from build123d import *

# Parameters (mm, degrees)
SKETCH1_W                                = 247.904
SKETCH1_H                                = 31.75
BOSS_EXTRUDE1_DEPTH                      = 5.9944
BOSS_EXTRUDE3_DEPTH                      = 5.9944
MIRROR2_AT_THE_SECOND_PLANE_COPY_1_DEPTH = 5.9944
SKETCH3_W                                = 12.7
SKETCH3_H                                = 2.9972
CUT_EXTRUDE1_DEPTH                       = 138.247848812


with BuildPart() as part:
    # Sketch1 → Boss-Extrude1 (new body)
    with BuildSketch(Plane(origin=(0, 0, 0), x_dir=(1, 0, 0), z_dir=(0, 1, 0))):
        Rectangle(SKETCH1_W, SKETCH1_H)
    extrude(amount=BOSS_EXTRUDE1_DEPTH)

    # Sketch4 → Boss-Extrude3 (add)
    with BuildSketch(Plane(origin=(0, 5.9944, 0), x_dir=(1, 0, 0), z_dir=(0, 1, 0))):
        Polygon((-123.952, 9.8806), (-136.1948, 9.8806), (-136.1948, 15.875), (-133.0198, 15.875), (-133.0198, 12.8778), (-129.8448, 12.8778), (-129.8448, 15.875), (-123.952, 15.875), align=None)
    boss_extrude3 = extrude(amount=-BOSS_EXTRUDE3_DEPTH)

    # Mirror2: Boss-Extrude3 across plane
    add(boss_extrude3.mirror(Plane.XY))

    # Mirror2 at the second plane: Boss-Extrude3 across plane
    add(boss_extrude3.mirror(Plane(origin=(0, 0, 0), x_dir=(0, 0, 1), z_dir=(1, 0, 0))))

    # Mirror2 at the second plane copy 1 sketc → Mirror2 at the second plane copy 1 (add)
    with BuildSketch(Plane(origin=(0, 5.9944, 0), x_dir=(-1, 0, 0), z_dir=(0, 1, 0))):
        Polygon((-123.952, 9.8806), (-136.1948, 9.8806), (-136.1948, 15.875), (-133.0198, 15.875), (-133.0198, 12.8778), (-129.8448, 12.8778), (-129.8448, 15.875), (-123.952, 15.875), align=None)
    extrude(amount=-MIRROR2_AT_THE_SECOND_PLANE_COPY_1_DEPTH)

    # Sketch3 → Cut-Extrude1 (cut, through all)
    with BuildSketch(Plane(origin=(0, 5.9944, 0), x_dir=(1, 0, 0), z_dir=(0, 1, 0))):
        with Locations((-74.3712, 0)):
            Rectangle(SKETCH3_W, SKETCH3_H)
        with Locations((-24.7904, 0)):
            Rectangle(SKETCH3_W, SKETCH3_H)
        with Locations((24.7904, 0)):
            Rectangle(SKETCH3_W, SKETCH3_H)
        with Locations((74.3712, 0)):
            Rectangle(SKETCH3_W, SKETCH3_H)
    extrude(amount=-CUT_EXTRUDE1_DEPTH, mode=Mode.SUBTRACT)


solid = part.part
Geometry check sheet. Reference: the model listing, model coordinates, mm. A direction names the side the tool comes from. Round coordinates to 2 decimals unless told otherwise and drop trailing zeros. Write each loop counter-clockwise with the first axis right and the second up, starting at its lowest first coordinate (ties: lowest second). Pieces come first, ordered by that corner, then holes.
Item 1: Go/stop test with flat-tipped pins: pin 1 Ø0.9 at (y, z) = (3.5, 0.5) entering from +X; pin 2 Ø1.5 at (x, z) = (-104, 4.5) entering from -Y; pin 3 Ø1 at (x, y) = (131, 4) entering from +Z; pin 4 Ø2.5 at (y, z) = (2, 0.5) entering from -X. Record where each tip stops, or that it passes through.
Determined:
pin 1: stops at x = 123.95
pin 2: stops at y = 0
pin 3: stops at z = 12.88
pin 4: stops at x = -123.95
Item 2: Material ranges on line 1 along X through (y, z) = (2, -0.5); line 2 along X through (y, z) = (2.3, 7); line 3 along Z through (x, y) = (-70, 0.5) (3 decimals), recorded low to high.
Determined:
line 1: x = -123.95 to -80.72, -68.02 to -31.14, -18.44 to 18.44, 31.14 to 68.02, 80.72 to 123.95
line 2: x = -123.95 to 123.95
line 3: z = -15.875 to -1.499, 1.499 to 15.875
Item 3: Access from +Z, -Z, +X, -X, +Y, -Y to the whole of each face (thin tool, end or side, straight path). Record for faces 5 (the face through (-25, 3, 1.499)), 6 (the face through (123.952, 3, 0)), 7 (the face through (-136.195, 3, -13)), 8 (the face through (-130, 3, 9.881)).
Determined:
face 5: +Y, -Y
face 6: +X, +Y, -Y
face 7: +Z, -Z, -X, +Y, -Y
face 8: -X, +Y, -Y
Item 4: Section check B-B (y = 2.9). Give the number of separate pieces and of enclosed holes in the cut face, plus the area to 3 significant figures.
Determined:
separate pieces: 1
enclosed holes: 4
area: 7,970 mm2
Item 5: Mould release check, pull along Z, two halves, no side actions. Record for faces 1 (the face through (2, 3, -15.875)), 2 (the face through (-74, 3, -1.499)), 3 (the face through (-130, 3, -9.881)), 4 (the face through (-2, 0, 0)): +Z half, -Z half, draft (parallel to the pull), parting line (faces both ways), or undercut.
Determined:
face 1: -Z half
face 2: undercut
face 3: undercut
face 4: draft
Item 6: Section check A-A (x = -23). Record the boundary of the cut face in (y, z) (3 decimals), plus the area to 3 significant figures.
Determined:
outline: (0, -15.875) - (5.994, -15.875) - (5.994, -1.499) - (0, -1.499) - close; (0, 1.499) - (5.994, 1.499) - (5.994, 15.875) - (0, 15.875) - close
area: 172 mm2
